Source: CAD feature listing. Evaluate the final solid. Frame: model axes, mm. A direction names the side the tool comes from. Round coordinates to 2 decimals unless told otherwise and drop trailing zeros. Write each loop counter-clockwise with the first axis right and the second up, starting at its lowest first coordinate (ties: lowest second). Pieces come first, ordered by that corner, then holes. Notation, with made-up numbers: (-13, 2.25) -> (30, 2.25) arc R24 cw to (30, 35.25) -> close; hole circle Ø8 at (8, 18.25). An arc over 180 degrees is marked (long way). Put each result on its own line as item: value.
```python
from build123d import *

# Parameters (mm, degrees)
BOSS_EXTRUDE1_START             = -30
SKETCH2_R                       = 11
BOSS_EXTRUDE1_DEPTH             = 1
BOSS_EXTRUDE1_DIRECTION_2_REACH = 73.569
SKETCH4_W                       = 7
SKETCH4_H                       = 7
BOSS_EXTRUDE2_DEPTH             = 6


with BuildPart() as part:
    # Sketch1 → Revolve-Thin1 (revolve)
    with BuildSketch(Plane.XY):
        with BuildLine():
            ThreePointArc((20, 0), (14.142135624, 14.142135624), (0, 20))
            Line((0, 20), (0, 24))
            ThreePointArc((0, 24), (16.970562748, 16.970562748), (24, 0))
            Line((24, 0), (20, 0))
        make_face()
    revolve(axis=Axis((0, 0, 0), (1, 0, 0)))

    # Sketch2 → Boss-Extrude1 (add)
    with BuildSketch(Plane.ZY.offset(BOSS_EXTRUDE1_START)):
        Circle(SKETCH2_R)
    extrude(amount=-BOSS_EXTRUDE1_DEPTH)

    # Sketch2 → Boss-Extrude1 direction 2 (add, up to next)
    with BuildSketch(Plane.ZY.offset(BOSS_EXTRUDE1_START), mode=Mode.PRIVATE) as boss_extrude1_direction_2_sk1:
        Circle(SKETCH2_R)
    boss_extrude1_direction_2_tool1 = extrude(boss_extrude1_direction_2_sk1.sketch, amount=BOSS_EXTRUDE1_DIRECTION_2_REACH, mode=Mode.PRIVATE) - part.part
    add(boss_extrude1_direction_2_tool1.solids().sort_by_distance((30, 0, 0))[0])

    # Sketch4 → Boss-Extrude2 (add)
    with BuildSketch(Plane(origin=(31, 0, 0), x_dir=(0, 0, -1), z_dir=(1, 0, 0))):
        Rectangle(SKETCH4_W, SKETCH4_H)
    extrude(amount=BOSS_EXTRUDE2_DEPTH)


solid = part.part
```
Q1. Cut plane C-C on x = 15.5. Output: boundary loops of the cut face in (y, z).
Ans:
outline: circle Ø36.65 at (0, 0); hole circle Ø25.28 at (0, 0)
Q2. Draft query along X for faces 4 (the flat face through (37, 0, 0)), 5 (the flat face through (34, 0, 3.5)), 6 (the flat face through (0, 5, 20)). Return one class per face: +X half, -X half, draft (parallel to the pull), parting line (faces both ways), or undercut.
Ans:
face 4: +X half
face 5: draft
face 6: -X half
Q3. Pin query (flat end, axial travel): pin 1 (5 mm diameter, centred on x = 35.5, z = -1.5, fed in from +Y); pin 2 (6.5 mm diameter, centred on x = 33, z = -1, fed in from -Y); pin 3 (5 mm diameter, centred on x = 33, y = 0.5, fed in from +Z); pin 4 (24 mm diameter, centred on y = 4.5, z = 1, fed in from +X). Return the tip coordinate at first contact, or that it passes through.
Ans:
pin 1: stops at y = 3.5
pin 2: stops at y = -11
pin 3: stops at z = 11
pin 4: stops at x = 37
Q4. Cut plane A-A on y = 0. Output: boundary loops of the cut face in (x, z).
Ans:
outline: (0, -24) arc R24 ccw to (21.33, -11) -> (31, -11) -> (31, -3.5) -> (37, -3.5) -> (37, 3.5) -> (31, 3.5) -> (31, 11) -> (21.33, 11) arc R24 ccw to (0, 24) -> (0, 20) arc R20 cw to (0, -20) -> close
Q5. Material intervals for line 1 (Y direction, x = 17, z = -5); line 2 (Z direction, x = 34, y = 0); line 3 (Y direction, x = 4.5, z = 9), sorted ascending. Write a range as [from, to].
Ans:
line 1: y = [-16.19, -9.27], [9.27, 16.19]
line 2: z = [-3.5, 3.5]
line 3: y = [-21.79, -17.28], [17.28, 21.79]
Q6. Reachability of faces 1 (the flat face through (34, 3.5, 0)), 2 (the flat face through (34, 0, -3.5)), 3 (the flat face through (34, -3.5, 0)) from +Z, -Z, +X, -X, +Y, -Y: full face, straight path, thin tool, end or side. Return the list, or none.
Ans:
face 1: +Z, -Z, +X, +Y
face 2: -Z, +X, +Y, -Y
face 3: +Z, -Z, +X, -Y
Q7. Cut plane D-D on z = 6. Output: boundary loops of the cut face in (x, y), and give its area (3 significant figures).
Ans:
outline: (0, -23.24) arc R23.24 ccw to (21.33, -9.22) -> (31, -9.22) -> (31, 9.22) -> (21.33, 9.22) arc R23.24 ccw to (0, 23.24) -> (0, 19.08) arc R19.08 cw to (0, -19.08) -> close
area: 431 mm^2
